Geometry: see drawing. Coordinates: mm, zero at the bounding-box minimum. Round coordinates to 2 decimals unless told otherwise and drop trailing zeros. Loops run counter-clockwise (first coordinate to the right, second up) from the corner with the lowest first, then second, coordinate; pieces in that order, holes last.
(1) First-contact query: pin 1 Ø1.2 at (y, z) = (2.5, 4) entering from +X; pin 2 Ø12 at (x, y) = (52.5, 32) entering from +Z; pin 3 Ø3 at (x, y) = (57, 26.5) entering from -Z; pin 4 Ø3 at (y, z) = (26, 3.5) entering from -X. Flat tips, straight axial feed; report the tip coordinate or a pass-through.
(2) Cut plane D-D, the plane z = 3.65. Output: boundary loops of the cut face in (x, y) (3 decimals), and give its area (3 significant figures).
(3) Cut plane B-B, the plane x = 37.5. Output: boundary loops of the cut face in (y, z), and give its area (3 significant figures).
(4) Cut plane C-C, the plane x = 13.5. Output: boundary loops of the cut face in (y, z).
(5) Line query: line 1 (X direction, y = 50.5, z = 2.6); line 2 (Z direction, x = 23.5, y = 18); line 3 (X direction, y = 16.5, z = 2.4). Output: solid intervals per line, ascending.
(6) Draft query along Y for the marked faces 1, 2 and 3. Return one class per face: released by +Y, released by -Y, zero draft, split by the parting line, or undercut.
(7) Cut plane A-A, the plane y = 33.5. Output: boundary loops of the cut face in (x, z).
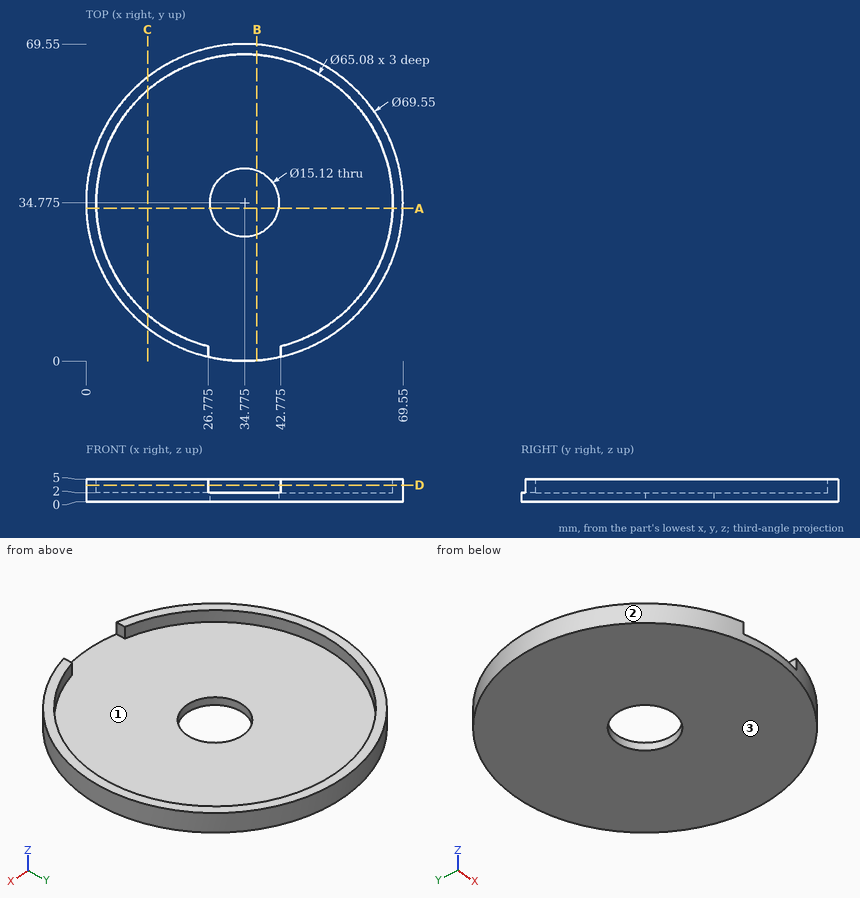
Reported:
1. pin 1: stops at x = 49.13
1. pin 2: stops at z = 2
1. pin 3: stops at z = 0
1. pin 4: stops at x = 0.77
2. outline: (26.775, 0.933) - (26.775, 3.234) arc R32.54 cw (long way) to (42.775, 3.234) - (42.775, 0.933) arc R34.775 ccw (long way) to start
2. area: 437 mm2
3. outline: (0.11, 0) - (27.72, 0) - (27.72, 2) - (0.11, 2) - close; (41.83, 0) - (69.44, 0) - (69.44, 5) - (67.2, 5) - (67.2, 2) - (41.83, 2) - close
3. area: 117 mm2
4. outline: (7.27, 0) - (62.28, 0) - (62.28, 5) - (59.4, 5) - (59.4, 2) - (10.15, 2) - (10.15, 5) - (7.27, 5) - close
5. line 1: x = 3.76 to 6.29, 63.26 to 65.79
5. line 2: z = 0 to 2
5. line 3: x = 5.19 to 7.85, 61.7 to 64.36
6. face 1: undercut
6. face 2: split by the parting line
6. face 3: zero draft
7. outline: (0.02, 0) - (27.32, 0) - (27.32, 2) - (2.26, 2) - (2.26, 5) - (0.02, 5) - close; (42.23, 0) - (69.53, 0) - (69.53, 5) - (67.29, 5) - (67.29, 2) - (42.23, 2) - close
